Build history of the part. All positions in model axes, mm. Face numbers are marked on the shaded views. A direction names the side the tool comes from. Round coordinates to 2 decimals unless told otherwise and drop trailing zeros. Order: outer loops, then holes, each group sorted by start corner. A loop starts at its lowest first (then second) coordinate and runs counter-clockwise, first axis right, second up. Notation, with made-up numbers: (24.5, -38.75) -> (30.5, -38.75) arc R17 cw to (30.5, -17.75) -> close; hole circle Ø8 at (88.25, -5.5). An arc over 180 degrees is marked (long way). Answer as CSV lines item,"result". Start each with the question number.
```python
from build123d import *

# Parameters (mm, degrees)
F3_DEPTH = 5
F5_DEPTH = 3


with BuildPart() as f1:
    # F0 (on Front) → F1 (revolve)
    with BuildSketch(Plane.XZ):
        Polygon((0, 16), (0, 0), (12.5, 0), (14, 4.5), (14, 12), (7.5, 16), align=None)
    revolve(axis=Axis((0, 0, 8), (0, 0, -1)))

    # F2 (on face) → F3 (cut)
    with BuildSketch(Plane.XY.offset(16)):
        with BuildLine():
            ThreePointArc((-1.941143, 7.244444), (0, 7.5), (1.941143, 7.244444))
            Line((1.941143, 7.244444), (3.623467, 13.522962))
            ThreePointArc((3.623467, 13.522962), (0, 14), (-3.623467, 13.522962))
            Line((-3.623467, 13.522962), (-1.941143, 7.244444))
        make_face()
        with BuildLine():
            ThreePointArc((-7.244444, 1.941143), (-6.495191, 3.75), (-5.303301, 5.303301))
            Line((-5.303301, 5.303301), (-9.899495, 9.899495))
            ThreePointArc((-9.899495, 9.899495), (-12.124356, 7), (-13.522962, 3.623467))
            Line((-13.522962, 3.623467), (-7.244444, 1.941143))
        make_face()
        with BuildLine():
            ThreePointArc((-5.303301, -5.303301), (-6.495191, -3.75), (-7.244444, -1.941143))
            Line((-7.244444, -1.941143), (-13.522962, -3.623467))
            ThreePointArc((-13.522962, -3.623467), (-12.124356, -7), (-9.899495, -9.899495))
            Line((-9.899495, -9.899495), (-5.303301, -5.303301))
        make_face()
        with BuildLine():
            ThreePointArc((1.941143, -7.244444), (0, -7.5), (-1.941143, -7.244444))
            Line((-1.941143, -7.244444), (-3.623467, -13.522962))
            ThreePointArc((-3.623467, -13.522962), (0, -14), (3.623467, -13.522962))
            Line((3.623467, -13.522962), (1.941143, -7.244444))
        make_face()
        with BuildLine():
            ThreePointArc((7.244444, -1.941143), (6.495191, -3.75), (5.303301, -5.303301))
            Line((5.303301, -5.303301), (9.899495, -9.899495))
            ThreePointArc((9.899495, -9.899495), (12.124356, -7), (13.522962, -3.623467))
            Line((13.522962, -3.623467), (7.244444, -1.941143))
        make_face()
        with BuildLine():
            ThreePointArc((5.303301, 5.303301), (6.495191, 3.75), (7.244444, 1.941143))
            Line((7.244444, 1.941143), (13.522962, 3.623467))
            ThreePointArc((13.522962, 3.623467), (12.124356, 7), (9.899495, 9.899495))
            Line((9.899495, 9.899495), (5.303301, 5.303301))
        make_face()
    extrude(amount=-F3_DEPTH, mode=Mode.SUBTRACT)

    # F4 (on face) → F5 (cut)
    with BuildSketch(Plane(origin=(0, 0, 0), x_dir=(1, 0, 0), z_dir=(0, 0, -1))):
        with BuildLine():
            ThreePointArc((2.911714, 10.866666), (7.954951, 7.954951), (10.866666, 2.911714))
            Line((10.866666, 2.911714), (13.522962, 3.623467))
            ThreePointArc((13.522962, 3.623467), (9.899495, 9.899495), (3.623467, 13.522962))
            Line((3.623467, 13.522962), (2.911714, 10.866666))
        make_face()
        with BuildLine():
            Line((-2.911714, 10.866666), (-3.623467, 13.522962))
            ThreePointArc((-3.623467, 13.522962), (-9.899495, 9.899495), (-13.522962, 3.623467))
            Line((-13.522962, 3.623467), (-10.866666, 2.911714))
            ThreePointArc((-10.866666, 2.911714), (-7.954951, 7.954951), (-2.911714, 10.866666))
        make_face()
        with BuildLine():
            Line((-10.866666, -2.911714), (-13.522962, -3.623467))
            ThreePointArc((-13.522962, -3.623467), (-9.899495, -9.899495), (-3.623467, -13.522962))
            Line((-3.623467, -13.522962), (-2.911714, -10.866666))
            ThreePointArc((-2.911714, -10.866666), (-7.954951, -7.954951), (-10.866666, -2.911714))
        make_face()
        with BuildLine():
            Line((2.911714, -10.866666), (3.623467, -13.522962))
            ThreePointArc((3.623467, -13.522962), (9.899495, -9.899495), (13.522962, -3.623467))
            Line((13.522962, -3.623467), (10.866666, -2.911714))
            ThreePointArc((10.866666, -2.911714), (7.954951, -7.954951), (2.911714, -10.866666))
        make_face()
    extrude(amount=-F5_DEPTH, mode=Mode.SUBTRACT)

    # F6 (on Front) → F7 (revolve)
    with BuildSketch(Plane.XZ):
        Polygon((0, 31), (0, 16), (7.5, 16), (7.7, 16.2), (7.7, 18.3), (7.5, 18.5), (2.5, 18.5), (2.5, 30.5), (2, 31), align=None)
    revolve(axis=Axis((0, 0, 23.5), (0, 0, -1)))


solid = f1.part
```
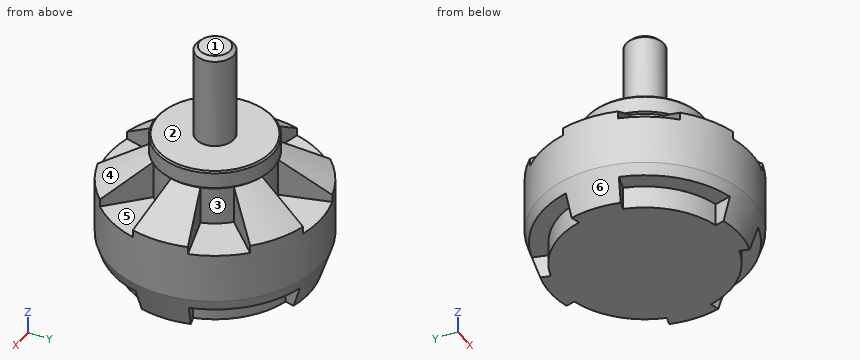
Q1. Slice it at B-B, the plane x = 0. Write the cut outline in (y, z), plus the area to 3 significant figures.
Q2. Slice it at D-D, the plane z = 8.5. Write the cut outline in (x, y), plus the area to 3 significant figures.
Q3. Slice it at A-A, the plane y = 0. Write the cut outline in (x, z).
Q4. Probe L1, parallel to Z at x = 4.75, y = 3.5; L2, parallel to Z at x = 5, y = -5.75; L3, parallel to Z at x = -9, y = 4.75. List the from-to ranges inside material, lowest first.
Q5. Two-plate mould, pull along X, no slides. Class the marked faces 4, 5 and 6: +X half, -X half, draft (parallel to the pull), parting line (faces both ways), or undercut.
Q6. Flat gauge pins, fed straight in: pin 1 Ø9 at (x, y) = (9.5, 8) entering from +Z; pin 2 Ø1 at (y, z) = (11, 5) entering from -X; pin 3 Ø3 at (x, y) = (-9, -7.5) entering from -Z; pin 4 Ø1.5 at (x, z) = (-3, 12) entering from +Y. Where does each tip first touch, or does it go through?
Q7. Slice it at C-C, the plane z = 21.5. Write the cut outline in (x, y).
Q8. Which spindle directions (+Z, -Z, +X, -X, +Y, -Y) get a long thin tool onto all of the face, cutting with end or side? Do the marked faces 1, 2 and 3. Say none if no direction does.
Solutions:
1,outline,"(-14, 4.5) -> (-12.5, 0) -> (12.5, 0) -> (14, 4.5) -> (14, 11) -> (7.5, 11) -> (7.5, 16) -> (7.7, 16.2) -> (7.7, 18.3) -> (7.5, 18.5) -> (2.5, 18.5) -> (2.5, 30.5) -> (2, 31) -> (-2, 31) -> (-2.5, 30.5) -> (-2.5, 18.5) -> (-7.5, 18.5) -> (-7.7, 18.3) -> (-7.7, 16.2) -> (-7.5, 16) -> (-7.5, 11) -> (-14, 11) -> close"
1,area,"477 mm2"
2,outline,"circle Ø28 at (0, 0)"
2,area,"616 mm2"
3,outline,"(-14, 4.5) -> (-12.5, 0) -> (12.5, 0) -> (14, 4.5) -> (14, 12) -> (7.5, 16) -> (7.7, 16.2) -> (7.7, 18.3) -> (7.5, 18.5) -> (2.5, 18.5) -> (2.5, 30.5) -> (2, 31) -> (-2, 31) -> (-2.5, 30.5) -> (-2.5, 18.5) -> (-7.5, 18.5) -> (-7.7, 18.3) -> (-7.7, 16.2) -> (-7.5, 16) -> (-14, 12) -> close"
4,L1,"z = 0 to 18.5"
4,L2,"z = 0 to 15.93, 16.12 to 18.38"
4,L3,"z = 0 to 11"
5,face 4,"+X half"
5,face 5,"undercut"
5,face 6,"parting line"
6,pin 1,"stops at z = 15.69"
6,pin 2,"stops at x = -9.26"
6,pin 3,"stops at z = 0"
6,pin 4,"stops at y = 13.52"
7,outline,"circle Ø5 at (0, 0)"
8,face 1,"+Z, +X, -X, +Y, -Y"
8,face 2,"+Z"
8,face 3,"none"
